Can you work these out from the model? Positions are in its coordinate system, mm. A direction names the side the tool comes from. Round coordinates to 2 decimals unless told otherwise and drop trailing zeros. Loops run counter-clockwise (first coordinate to the right, second up) from the corner with the lowest first, then second, coordinate; pieces in that order, holes last. Notation, with made-up numbers: M 88.25,85 L 129.25,85 A16 ccw 129.25,95 Z; hole C 5.25,87.25 d1. An arc over 180 degrees is marked long. Return JSON: item names as keys, results as strings.
Autodesk Inventor part; units mm, degrees
ref_plane "YZ Plane" through (0, 0, 0) normal (1, 0, 0) x (0, 1, 0)
ref_plane "XZ Plane" through (0, 0, 0) normal (0, 1, 0) x (-1, 0, 0)
ref_plane "XY Plane" through (0, 0, 0) normal (0, 0, 1) x (1, 0, 0)
sketch "Skizze4" plane through (0, 0, 0) normal (0, 1, 0) x (-1, 0, 0)
  line L0 (-33.6472, -5.1972) -> (-47.1472, -5.1972)
  line L1 (-47.1472, -5.1972) -> (-47.1472, -7.0972)
  line L2 (-47.1472, -7.0972) -> (-47.1472, -7.0972)
  line L3 (-47.1472, -7.0972) -> (-47.1472, -8.2972)
  line L4 (-47.1472, -8.2972) -> (-47.1472, -8.2972)
  line L5 (-47.1472, -8.2972) -> (-47.1472, -10.1972)
  line L6 (-47.1472, -10.1972) -> (-33.6472, -10.1972)
  line L7 (-33.6472, -10.1972) -> (-33.6472, -8.2972)
  line L8 (-33.6472, -8.2972) -> (-33.6472, -8.2972)
  line L9 (-33.6472, -8.2972) -> (-33.6472, -7.0972)
  line L10 (-33.6472, -7.0972) -> (-33.6472, -7.0972)
  line L11 (-33.6472, -7.0972) -> (-33.6472, -5.1972)
  dimension "Kerbentiefe" = 0
  dimension "b_Halter" = 13.5
  dimension "d12" = 0
  dimension "Kerbenbreite" = 1.2
  dimension "d_Halter" = 5
extrude "Extrusion3" add sketch "Skizze4" along normal blind 70
sketch "Skizze6" plane through (33.6472, 0, -5.1972) normal (0, 0, 1) x (1, 0, 0)
  line L0 (0, 70) -> (13.5, 70)
  line L1 (0.75, 68.1) -> (11.95, 68.1)
  line L2 (11.95, 68.1) -> (11.95, 57.4)
  line L3 (11.95, 57.4) -> (0.75, 57.4)
  line L4 (0.75, 57.4) -> (0.75, 68.1)
  line L5 (0, 0) -> (13.5, 0)
  line L6 (6.75, 70) -> (6.75, 0) construction
  dimension "d20" = 1.9
  dimension "d21" = 10.7
  dimension "d22" = 11.2
  dimension "d31" = 5.2
extrude "Extrusion5" cut sketch "Skizze6" against normal blind 0.5
sketch "Skizze7" plane through (33.6472, 0, -5.1972) normal (0, 0, 1) x (1, 0, 0)
  line L0 (0.75, 68.1) -> (11.95, 68.1)
  line L1 (0, 0) -> (13.5, 0)
  line L2 (0.75, 68.1) -> (11.95, 68.1)
  line L3 (4.85, 68.1) -> (7.85, 68.1)
  line L4 (7.85, 68.1) -> (7.85, 0)
  line L5 (7.85, 0) -> (4.85, 0)
  line L6 (4.85, 0) -> (4.85, 68.1)
  line L7 (0.75, 57.4) -> (0.75, 68.1)
  dimension "d26" = 3
  dimension "d32" = 4.1
extrude "Extrusion6" cut sketch "Skizze7" against normal blind 2
ref_plane "hor_Strahlebene" through (34.3972, 62.75, -5.1972) normal (0, 1, 0) x (1, 0, 0)
ref_plane "Ebene_Anschlag2" through (34.3972, 11.75, -5.1972) normal (0, 1, 0) x (1, 0, 0)
sketch "Skizze10" plane through (0, 0, 0) normal (0, -1, 0) x (1, 0, 0)
  line L0 (33.6472, -5.1972) -> (32.6472, -5.1972)
  line L1 (32.6472, -5.1972) -> (32.6472, -10.1972)
  line L2 (32.6472, -10.1972) -> (33.6472, -10.1972)
  line L3 (33.6472, -10.1972) -> (33.6472, -5.1972)
  dimension "d36" = 1
extrude "Extrusion8" add sketch "Skizze10" against normal up to surface (11.75 mm away)
ref_plane "Mittelebene_Halter" through (40.3972, 70, -10.1972) normal (-1, 0, 0) x (0, 0, 1)
mirror "Spiegeln1" about plane through (40.3972, 70, -10.1972) normal (-1, 0, 0) of "Extrusion8"
ref_plane "Arbeitsebene4" through (40.3972, 70, -10.1972) normal (-1, 0, 0) x (0, 0, 1)
equation "\"d32\" = -0.5 * d26 + 0.5 * d22"
properties part number "Halter_PP" material "ABS-Kunststoff"
Q1. Suppose I cut it at B-B, the plane z = -8. Please give me the cut outline in (x, y).
Results:
{"outline": "M 32.65,0 L 48.15,0 L 48.15,11.75 L 47.15,11.75 L 47.15,70 L 33.65,70 L 33.65,11.75 L 32.65,11.75 Z"}
Q2. If I drill on line 1 along X through (y, z) = (14.5, -5.85); line 2 along X through (y, z) = (36, -7.6); line 3 along Z through (x, y) = (39, 21.5), over which ranges is the centre line in solid material (lowest first)?
Results:
{"line 1": "x = 33.65 to 38.5, 41.5 to 47.15", "line 2": "x = 33.65 to 47.15", "line 3": "z = -10.2 to -7.2"}
Q3. I'm going to push flat-ended pins straight in: pin 1 Ø3.5 at (x, y) = (40.5, 26) entering from +Z; pin 2 Ø1.6 at (y, z) = (37, -6.5) entering from +X; pin 3 Ø2 at (y, z) = (23, -6) entering from -X; pin 4 Ø4.5 at (x, y) = (43, 63.5) entering from +Z. Where does each tip first touch, or does it pass through?
Results:
{"pin 1": "stops at z = -5.2", "pin 2": "stops at x = 47.15", "pin 3": "stops at x = 33.65", "pin 4": "stops at z = -5.7"}
Q4. On a 3-axis mill with a long thin cutter (end or side, diameter ignored), from which of +Z, -Z, +X, -X, +Y, -Y can I reach the whole of each face in a straight line? I mean faces 1 (the flat face through (47.147, 40, -8)), 2 (the flat face through (40, 35, -7.197)), 3 (the flat face through (36, 63, -5.697)). Say none if no direction works.
Results:
{"face 1": "+Z, -Z, +X, +Y", "face 2": "+Z, -Y", "face 3": "+Z"}
Q5. Suppose I cut it at A-A, the plane y = 46. Please give me the cut outline in (x, z), plus the area to 3 significant figures.
Results:
{"outline": "M 33.65,-10.2 L 47.15,-10.2 L 47.15,-5.2 L 41.5,-5.2 L 41.5,-7.2 L 38.5,-7.2 L 38.5,-5.2 L 33.65,-5.2 Z", "area": "61.5 mm2"}
Q6. Suppose I cut it at C-C, the plane x = 39.5. Please give me the cut outline in (y, z).
Results:
{"outline": "M 0,-10.2 L 70,-10.2 L 70,-5.2 L 68.1,-5.2 L 68.1,-7.2 L 0,-7.2 Z"}
Q7. Suppose I cut it at D-D, the plane y = 59. Please give me the cut outline in (x, z), plus the area to 3 significant figures.
Results:
{"outline": "M 33.65,-10.2 L 47.15,-10.2 L 47.15,-5.2 L 45.6,-5.2 L 45.6,-5.7 L 41.5,-5.7 L 41.5,-7.2 L 38.5,-7.2 L 38.5,-5.7 L 34.4,-5.7 L 34.4,-5.2 L 33.65,-5.2 Z", "area": "57.4 mm2"}
Q8. Thinking about a two-plate mould opening in Y: for faces 4 (the flat face through (40, 70, -8)), 5 (the flat face through (42, 27, -5.197)), 6 (the flat face through (40, 68.1, -6)), which applies, pulls with the +Y half, pulls with the -Y half, needs draft (parallel to the pull), parting line crosses it, or undercut?
Results:
{"face 4": "pulls with the +Y half", "face 5": "needs draft", "face 6": "undercut"}
